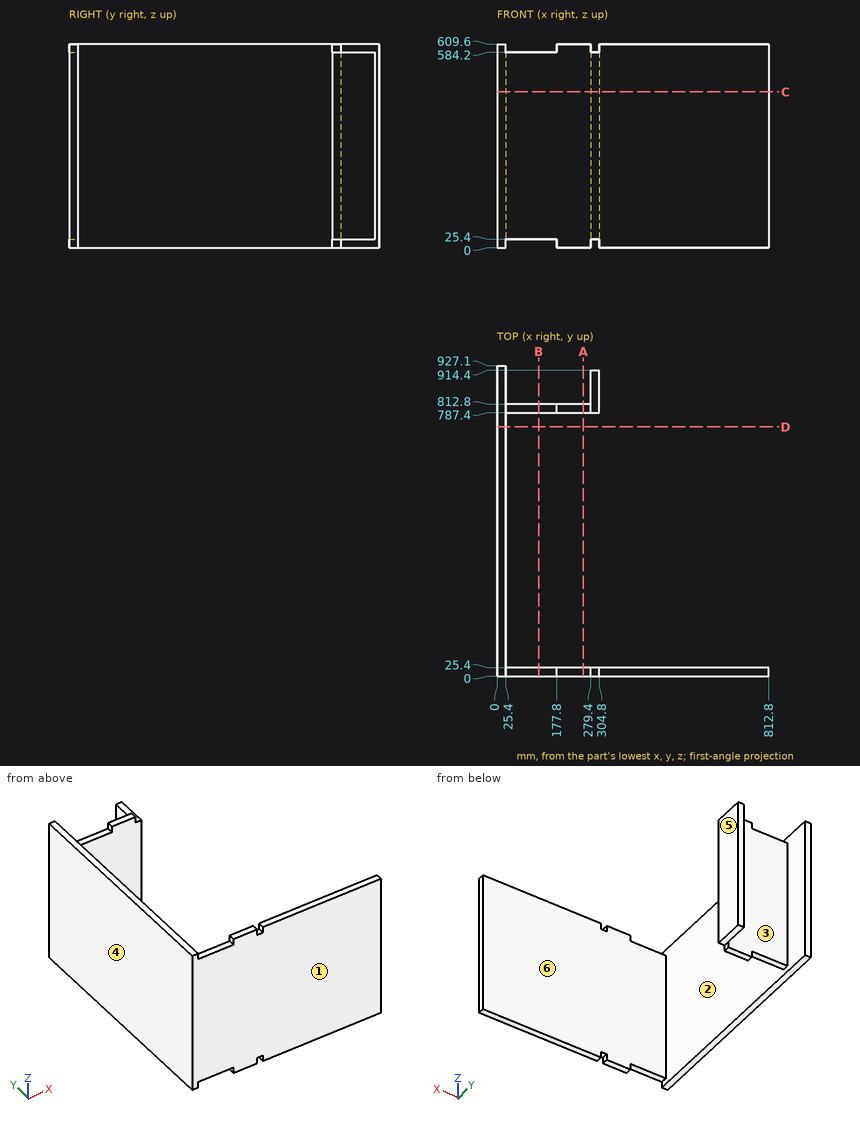
Here's the drawing with two shaded views (mm, measured from the low corner). I have some questions. A direction names the side the tool comes from. Round coordinates to 2 decimals unless told otherwise and drop trailing zeros. Order: outer loops, then holes, each group sorted by start corner. A loop starts at its lowest first (then second) coordinate and runs counter-clockwise, first axis right, second up. Notation, with made-up numbers: M 84,22.25 L 143,22.25 A17 ccw 143,45.25 Z; hole C -36.75,-40 d2. An arc over 180 degrees is marked long. Answer in a Markdown table with one row per item.
Item 1: Imagine slicing it at B-B, the plane x = 124. Write out the boundary of the cut face in (y, z), and give its area (3 significant figures).
A:
| item | result |
|---|---|
| outline | M 0,25.4 L 25.4,25.4 L 25.4,584.2 L 0,584.2 Z; M 787.4,25.4 L 812.8,25.4 L 812.8,584.2 L 787.4,584.2 Z |
| area | 28,400 mm2 |
Item 2: If I drill on L1, parallel to X at y = 839, z = 63; L2, parallel to Y at x = 282.5, z = 54.5; L3, parallel to Y at x = 85.5, z = 531.5, over which ranges is the centre line in solid material (lowest first)? Write a range as from..to.
A:
| item | result |
|---|---|
| L1 | x = 0..25.4, 279.4..304.8 |
| L2 | y = 0..25.4, 787.4..914.4 |
| L3 | y = 0..25.4, 787.4..812.8 |
Item 3: For the marked faces 5 and 6, which set-ups out of +Z, -Z, +X, -X, +Y, -Y let a thin tool reach every point of the face, with its end or its side?
A:
| item | result |
|---|---|
| face 5 | +Z, -Z, +X, +Y |
| face 6 | +Z, -Z, +X |
Item 4: Imagine slicing it at D-D, the plane y = 745. Write out the boundary of the cut face in (x, z), and give its area (3 significant figures).
A:
| item | result |
|---|---|
| outline | M 0,0 L 25.4,0 L 25.4,609.6 L 0,609.6 Z |
| area | 15,500 mm2 |
Item 5: Imagine slicing it at C-C, the plane z = 466.5. Write out the boundary of the cut face in (x, y), and give its area (3 significant figures).
A:
| item | result |
|---|---|
| outline | M 0,0 L 812.8,0 L 812.8,25.4 L 25.4,25.4 L 25.4,787.4 L 304.8,787.4 L 304.8,914.4 L 279.4,914.4 L 279.4,812.8 L 25.4,812.8 L 25.4,927.1 L 0,927.1 Z |
| area | 53,200 mm2 |
Item 6: I'm going to push flat-ended pins straight in: pin 1 (5 mm diameter, centred on y = 255, z = 128, fed in from +X); pin 2 (6 mm diameter, centred on x = 287, z = 291, fed in from -Y); pin 3 (7.5 mm diameter, centred on y = 805.5, z = 13, fed in from +X); pin 4 (7.5 mm diameter, centred on x = 294, y = 836, fed in from +Z). Where does each tip first touch, or does it pass through?
A:
| item | result |
|---|---|
| pin 1 | stops at x = 25.4 |
| pin 2 | stops at y = 0 |
| pin 3 | stops at x = 279.4 |
| pin 4 | stops at z = 584.2 |
Item 7: Imagine slicing it at A-A, the plane x = 258. Write out the boundary of the cut face in (y, z), and give its area (3 significant figures).
A:
| item | result |
|---|---|
| outline | M 0,0 L 25.4,0 L 25.4,609.6 L 0,609.6 Z; M 787.4,0 L 812.8,0 L 812.8,609.6 L 787.4,609.6 Z |
| area | 31,000 mm2 |
Item 8: Thinking about a two-plate mould opening in Y: for the marked faces 1, 2, 3 and 4, which applies, +Y half, -Y half, draft (parallel to the pull), parting line (faces both ways), or undercut?
A:
| item | result |
|---|---|
| face 1 | -Y half |
| face 2 | undercut |
| face 3 | +Y half |
| face 4 | draft |
